```python
from build123d import *

# Parameters (mm, degrees)
SKETCH_5_W          = 64
SKETCH_5_H          = 140
EXTRUDE_4_DEPTH     = 2.75
SKETCH_6_R          = 1.7
CUT_EXTRUDE_1_DEPTH = 8
CUT_EXTRUDE_2_DEPTH = 10


with BuildPart() as part:
    # 草图5 → 凸台-拉伸4 (new, symmetric)
    with BuildSketch(Plane(origin=(0, 0, 0), x_dir=(1, 0, 0), z_dir=(0, 1, 0))):
        Rectangle(SKETCH_5_W, SKETCH_5_H)
    extrude(amount=EXTRUDE_4_DEPTH, both=True)

    # 草图6 → 切除-拉伸1 (cut)
    with BuildSketch(Plane(origin=(0, 2.75, 0), x_dir=(1, 0, 0), z_dir=(0, 1, 0))):
        with Locations(Location((-24, 65, 0), (0, 0, 270))):
            Circle(SKETCH_6_R)
        with Locations(Location((-24, -65, 0), (0, 0, 90))):
            Circle(SKETCH_6_R)
        with Locations(Location((24, -65, 0), (0, 0, 270))):
            Circle(SKETCH_6_R)
        with Locations(Location((24, 65, 0), (0, 0, 90))):
            Circle(SKETCH_6_R)
        with Locations(Location((-14, 65, 0), (0, 0, 270))):
            Circle(SKETCH_6_R)
        with Locations(Location((-14, -65, 0), (0, 0, 90))):
            Circle(SKETCH_6_R)
        with Locations(Location((14, -65, 0), (0, 0, 270))):
            Circle(SKETCH_6_R)
        with Locations(Location((14, 65, 0), (0, 0, 90))):
            Circle(SKETCH_6_R)
    extrude(amount=-CUT_EXTRUDE_1_DEPTH, mode=Mode.SUBTRACT)

    # 草图7 → 切除-拉伸2 (cut)
    with BuildSketch(Plane(origin=(0, 2.75, 0), x_dir=(1, 0, 0), z_dir=(0, 1, 0))):
        with BuildLine():
            Line((-10.893389513, 40), (-10.893389513, -40))
            ThreePointArc((-10.893389513, -40), (-14.893389513, -44), (-18.893389513, -40))
            Line((-18.893389513, -40), (-18.893389513, 40))
            ThreePointArc((-18.893389513, 40), (-14.893389513, 44), (-10.893389513, 40))
        make_face()
        with BuildLine():
            Line((10.893389513, 40), (10.893389513, -40))
            ThreePointArc((10.893389513, -40), (14.893389513, -44), (18.893389513, -40))
            Line((18.893389513, -40), (18.893389513, 40))
            ThreePointArc((18.893389513, 40), (14.893389513, 44), (10.893389513, 40))
        make_face()
    extrude(amount=-CUT_EXTRUDE_2_DEPTH, mode=Mode.SUBTRACT)


solid = part.part
```
Can you work these out from the model? Positions are in its coordinate system, mm. A direction names the side the tool comes from. Give positions to 0.01 mm unless a question says otherwise; leave off trailing zeros. Write each loop counter-clockwise with the first axis right and the second up, starting at its lowest first coordinate (ties: lowest second). Pieces come first, ordered by that corner, then holes. Notation, with made-up numbers: (76, 30) - (86, 30) arc R10 cw to (86, 35) - close; hole circle Ø7 at (-24.75, 17.25). An arc over 180 degrees is marked (long way). Write item = value, one per line. Start each with the question number.
1. Imagine slicing it at A-A (z = 65). Please give me the cut outline in (x, y).
2. Imagine slicing it at B-B (y = 0.15). Count the separate pieces of the cut face and the enclosed holes in it, and give its area (3 significant figures).
3. On a 3-axis mill with a long thin cutter (end or side, diameter ignored), from which of +Z, -Z, +X, -X, +Y, -Y can I reach the whole of each face in a straight line? I mean faces 1 (the face through (-15, 0, -44)), 2 (the face through (0, 0, 70)). Say none if no direction works.
4. For pin 1 (2 mm diameter, centred on x = 24, z = -65, fed in from +Y), with a flat end and sliding along its axis, tell me the tip position at first contact or that it passes through.
5. Imagine slicing it at D-D (z = -4). Please give me the cut outline in (x, y), and give its area (3 significant figures).
6. Thinking about a two-plate mould opening in Z: for faces 3 (the face through (-15, 0, 44)), 4 (the face through (0, -2.75, -1)), 5 (the face through (0, 0, -70)), which applies, released by +Z, released by -Z, zero draft, split by the parting line, or undercut?
7. Please list where these lines run through material, in increasing order: line 1 (X direction, y = 0, z = 35); line 2 (X direction, y = -1.25, z = 65); line 3 (Z direction, x = -13, y = -1.3).
8. Imagine slicing it at C-C (x = 24). Please give me the cut outline in (y, z), and give its area (3 significant figures).
Worked answers:
q1.outline = (-32, -2.75) - (-25.7, -2.75) - (-25.7, 2.75) - (-32, 2.75) - close; (-22.3, -2.75) - (-15.7, -2.75) - (-15.7, 2.75) - (-22.3, 2.75) - close; (-12.3, -2.75) - (12.3, -2.75) - (12.3, 2.75) - (-12.3, 2.75) - close; (15.7, -2.75) - (22.3, -2.75) - (22.3, 2.75) - (15.7, 2.75) - close; (25.7, -2.75) - (32, -2.75) - (32, 2.75) - (25.7, 2.75) - close
q2.separate_pieces = 1
q2.enclosed_holes = 10
q2.area = 7,510 mm2
q3.face_1 = +Y, -Y
q3.face_2 = +Z, +X, -X, +Y, -Y
q4.pin_1 = through
q5.outline = (-32, -2.75) - (-18.89, -2.75) - (-18.89, 2.75) - (-32, 2.75) - close; (-10.89, -2.75) - (10.89, -2.75) - (10.89, 2.75) - (-10.89, 2.75) - close; (18.89, -2.75) - (32, -2.75) - (32, 2.75) - (18.89, 2.75) - close
q5.area = 264 mm2
q6.face_3 = undercut
q6.face_4 = zero draft
q6.face_5 = released by -Z
q7.line_1 = -32 to -18.89, -10.89 to 10.89, 18.89 to 32
q7.line_2 = -32 to -25.7, -22.3 to -15.7, -12.3 to 12.3, 15.7 to 22.3, 25.7 to 32
q7.line_3 = -70 to -66.37, -63.63 to -43.52, 43.52 to 63.63, 66.37 to 70
q8.outline = (-2.75, -70) - (2.75, -70) - (2.75, -66.7) - (-2.75, -66.7) - close; (-2.75, -63.3) - (2.75, -63.3) - (2.75, 63.3) - (-2.75, 63.3) - close; (-2.75, 66.7) - (2.75, 66.7) - (2.75, 70) - (-2.75, 70) - close
q8.area = 733 mm2
